Could you check a few things on this model? Use its own coordinates, in mm. Coordinates: 2 decimals unless noted, no trailing zeros. Loops run counter-clockwise (first coordinate to the right, second up) from the corner with the lowest first, then second, coordinate; pieces in that order, holes last.
from build123d import *

# Parameters (mm, degrees)
SKETCH2_W           = 500
SKETCH2_H           = 100.85
BOSS_EXTRUDE1_DEPTH = 12
SKETCH4_W           = 12
SKETCH4_H           = 12
CUT_EXTRUDE2_DEPTH  = 511.210468826
SKETCH5_W           = 166.666666666
SKETCH5_H           = 12
CUT_EXTRUDE3_DEPTH  = 511.210468826
SCALE1_SCALE        = 0.5


with BuildPart() as part:
    # Sketch2 → Boss-Extrude1 (new body)
    with BuildSketch(Plane(origin=(0, 0, 0), x_dir=(1, 0, 0), z_dir=(0, 1, 0))):
        with Locations((250, 50.425)):
            Rectangle(SKETCH2_W, SKETCH2_H)
    extrude(amount=BOSS_EXTRUDE1_DEPTH)

    # Sketch4 → Cut-Extrude2 (cut, through all)
    with BuildSketch(Plane(origin=(0, 12, 0), x_dir=(1, 0, 0), z_dir=(0, 1, 0))):
        with Locations((494, 6)):
            Rectangle(SKETCH4_W, SKETCH4_H)
        with Locations((494, 94.85)):
            Rectangle(SKETCH4_W, SKETCH4_H)
        with Locations((6, 94.85)):
            Rectangle(SKETCH4_W, SKETCH4_H)
        with Locations((6, 6)):
            Rectangle(SKETCH4_W, SKETCH4_H)
    extrude(amount=-CUT_EXTRUDE2_DEPTH, mode=Mode.SUBTRACT)

    # Sketch5 → Cut-Extrude3 (cut, through all)
    with BuildSketch(Plane(origin=(0, 12, 0), x_dir=(1, 0, 0), z_dir=(0, 1, 0))):
        with Locations((250, 94.85)):
            Rectangle(SKETCH5_W, SKETCH5_H)
        with Locations((250, 6)):
            Rectangle(SKETCH5_W, SKETCH5_H)
    extrude(amount=-CUT_EXTRUDE3_DEPTH, mode=Mode.SUBTRACT)


with BuildPart() as part_1:
    # Scale1: scaled about (250, 6, -50.425)
    add(part.part.scale(SCALE1_SCALE).moved(Location((125, 3, -25.2125))))


solid = part_1.part
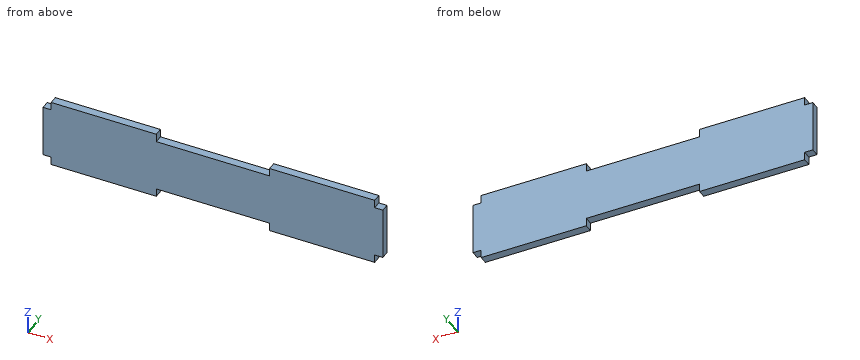
(1) Imagine slicing it at B-B, the plane x = 226.5. Write out the boundary of the cut face in (y, z), and give its area (3 significant figures).
Answers:
outline: (3, -69.64) - (9, -69.64) - (9, -31.21) - (3, -31.21) - close
area: 231 mm2
(2) For pin 1 (3 mm diameter, centred on y = 7, z = -27.5, fed in from -X); pin 2 (1.8 mm diameter, centred on x = 128.5, y = 6, fed in from +Z); pin 3 (3 mm diameter, centred on x = 243.5, y = 5, fed in from -Z), each with a flat end and sliding along its axis, tell me the tip position at first contact or that it passes through.
Answers:
pin 1: stops at x = 131
pin 2: stops at z = -31.21
pin 3: stops at z = -69.64
(3) Imagine slicing it at A-A, the plane y = 7.85. Write out the boundary of the cut face in (x, z), and give its area (3 significant figures).
Answers:
outline: (125, -69.64) - (131, -69.64) - (131, -75.64) - (208.33, -75.64) - (208.33, -69.64) - (291.67, -69.64) - (291.67, -75.64) - (369, -75.64) - (369, -69.64) - (375, -69.64) - (375, -31.21) - (369, -31.21) - (369, -25.21) - (291.67, -25.21) - (291.67, -31.21) - (208.33, -31.21) - (208.33, -25.21) - (131, -25.21) - (131, -31.21) - (125, -31.21) - close
area: 11,500 mm2
(4) I need wall thicknesses on probe 1 along X at (y, z) = (7.7, -71.5); probe 2 along Z at (x, y) = (253, 6). Which ranges of each line are inside material? Lowest first, please.
Answers:
probe 1: x = 131 to 208.33, 291.67 to 369
probe 2: z = -69.64 to -31.21
